```python
from build123d import *

# Parameters (mm, degrees)
ESTRUSIONE_ESTRUSIONE1_DEPTH = 2
CROQUIS2_R                   = 2
CROQUIS2_W                   = 40.7
CROQUIS2_H                   = 20
CORTAR_EXTRUIR1_DEPTH        = 59.660037504


with BuildPart() as part:
    # Schizzo1 → Estrusione-Estrusione1 (new, symmetric)
    with BuildSketch(Plane(origin=(0, 0, 0), x_dir=(1, 0, 0), z_dir=(0, 1, 0))):
        with BuildLine():
            Line((-25, 37.416573868), (-25, 27.25))
            Line((-25, 27.25), (25, 27.25))
            Line((25, 27.25), (25, 37.416573868))
            ThreePointArc((25, 37.416573868), (45, 0), (25, -37.416573868))
            Line((25, -37.416573868), (25, -27.25))
            Line((25, -27.25), (-25, -27.25))
            Line((-25, -27.25), (-25, -37.416573868))
            ThreePointArc((-25, -37.416573868), (-45, 0), (-25, 37.416573868))
        make_face()
    extrude(amount=ESTRUSIONE_ESTRUSIONE1_DEPTH, both=True)

    # Croquis2 → Cortar-Extruir1 (cut, through all)
    with BuildSketch(Plane(origin=(0, 2, 0), x_dir=(1, 0, 0), z_dir=(0, 1, 0))):
        with Locations(Location((-34.7, 5, 0), (0, 0, 270))):
            Circle(CROQUIS2_R)
        with Locations(Location((-34.7, -5, 0), (0, 0, 270))):
            Circle(CROQUIS2_R)
        with Locations(Location((14, 5, 0), (0, 0, 270))):
            Circle(CROQUIS2_R)
        with Locations(Location((14, -5, 0), (0, 0, 270))):
            Circle(CROQUIS2_R)
        with Locations(Location((0, 21.25, 0), (0, 0, 270))):
            Circle(CROQUIS2_R)
        with Locations(Location((0, -21.25, 0), (0, 0, 270))):
            Circle(CROQUIS2_R)
        with Locations((-10.35, 0)):
            Rectangle(CROQUIS2_W, CROQUIS2_H)
    extrude(amount=-CORTAR_EXTRUIR1_DEPTH, mode=Mode.SUBTRACT)


solid = part.part
```
The listing builds one solid part. Answer for the finished solid, in the listing's coordinates (mm). A direction names the side the tool comes from. Coordinates: 2 decimals unless noted, no trailing zeros. Write each loop counter-clockwise with the first axis right and the second up, starting at its lowest first coordinate (ties: lowest second). Pieces come first, ordered by that corner, then holes. Notation, with made-up numbers: (36.5, 50) - (44.5, 50) arc R25 ccw to (44.5, 73) - close; hole circle Ø3 at (43, 4.25). An arc over 180 degrees is marked (long way). Return JSON: item names as keys, results as strings. Group by question number.
1. Given pin 1 (1 mm diameter, centred on y = -1.5, z = 3.5, fed in from +X); pin 2 (6.5 mm diameter, centred on x = -34.7, z = 5, fed in from +Y); pin 3 (1.2 mm diameter, centred on x = -8, y = 1, fed in from +Z); pin 4 (2 mm diameter, centred on x = -11, y = 0.5, fed in from -Z), each flat-ended and moving along its own axis, determine where each tip first touches the part or whether it passes through.
2. Straight lines are drawn through the part: L1, parallel to Z at x = -20, y = -1.2; L2, parallel to Z at x = -36, y = -0.65; L3, parallel to X at y = -0.4, z = -1. For each, find the intervals that lie inside material, in ascending order.
3. A cutting plane is placed at D-D, the plane z = 33.5. Determine the outline of the cut face in (x, y), plus the area to 3 significant figures.
4. Which of the six approach directions +Z, -Z, +X, -X, +Y, -Y give full straight-line access (tool end or side, diameter ignored) to faces 1 (the cylindrical face through (-44.996, 0.028, 0.618)), 2 (the flat face through (25, 0, 32)), 3 (the flat face through (10, 0, 0)), 4 (the flat face through (-25, 0, -32))?
5. Determine the mould class of faces 5 (the cylindrical face through (44.996, 0.028, -0.618)), 6 (the flat face through (11, 2, -1)), 7 (the flat face through (-30.7, 0, 0)) for opening direction X: released by +X, released by -X, zero draft, split by the parting line, or undercut.
6. A cutting plane is placed at C-C, the plane y = 1.15. Determine the outline of the cut face in (x, z), plus the area to 3 significant figures.
7. A cutting plane is placed at A-A, the plane x = -23. Determine the outline of the cut face in (y, z), plus the area to 3 significant figures.
8. A cutting plane is placed at B-B, the plane x = 0. Determine the outline of the cut face in (y, z), plus the area to 3 significant figures.
Ans:
{
 "1": {"pin 1": "x = 44.9", "pin 2": "y = 2", "pin 3": "z = 27.25", "pin 4": "z = -27.25"},
 "2": {"L1": "-27.25 to -10, 10 to 27.25", "L2": "-27 to -6.52, -3.48 to 3.48, 6.52 to 27", "L3": "-44.99 to -30.7, 10 to 44.99"},
 "3": {"outline": "(-30.05, -2) - (-25, -2) - (-25, 2) - (-30.05, 2) - close; (25, -2) - (30.05, -2) - (30.05, 2) - (25, 2) - close", "area": "40.4 mm²"},
 "4": {"face 1": "-X, +Y, -Y", "face 2": "+Z, +Y, -Y", "face 3": "+Y, -Y", "face 4": "-Z, +Y, -Y"},
 "5": {"face 5": "released by +X", "face 6": "zero draft", "face 7": "undercut"},
 "6": {"outline": "(-25, -37.42) - (-25, -27.25) - (25, -27.25) - (25, -37.42) arc R45 ccw to (25, 37.42) - (25, 27.25) - (-25, 27.25) - (-25, 37.42) arc R45 ccw to start; hole circle Ø4 at (-34.7, -5); hole circle Ø4 at (-34.7, 5); hole (-30.7, -10) - (10, -10) - (10, 10) - (-30.7, 10) - close; hole circle Ø4 at (0, -21.25); hole circle Ø4 at (0, 21.25); hole circle Ø4 at (14, -5); hole circle Ø4 at (14, 5)", "area": "3,940 mm²"},
 "7": {"outline": "(-2, -27.25) - (2, -27.25) - (2, -10) - (-2, -10) - close; (-2, 10) - (2, 10) - (2, 27.25) - (-2, 27.25) - close", "area": "138 mm²"},
 "8": {"outline": "(-2, -27.25) - (2, -27.25) - (2, -23.25) - (-2, -23.25) - close; (-2, -19.25) - (2, -19.25) - (2, -10) - (-2, -10) - close; (-2, 10) - (2, 10) - (2, 19.25) - (-2, 19.25) - close; (-2, 23.25) - (2, 23.25) - (2, 27.25) - (-2, 27.25) - close", "area": "106 mm²"}
}
